For this review, take the finished solid that the model builds, in its own axes (mm). Face numbers are marked on the shaded views. A direction names the side the tool comes from. Round coordinates to 2 decimals unless told otherwise and drop trailing zeros. Write each loop counter-clockwise with the first axis right and the second up, starting at its lowest first coordinate (ties: lowest second). Pieces come first, ordered by that corner, then holes. Notation, with made-up numbers: (3, 49) - (16, 49) arc R24 cw to (16, 88) - close; hole circle Ø4 at (-9, 67.25). An arc over 180 degrees is marked (long way). One line per item, written item: value. Start each with the question number.
Q1. Mouldability with a two-part tool opening along Z and no side actions: class the marked faces 6, 7 and 8 as +Z half, -Z half, draft (parallel to the pull), parting line (faces both ways), or undercut.
Q2. Clearance check with flat-ended pins moving along their axes: pin 1 Ø4 at (x, z) = (3.5, 7) entering from -Y; pin 2 Ø3 at (y, z) = (1, 0) entering from -X; pin 3 Ø2 at (y, z) = (-5, -2.5) entering from +X. State where each tip first meets the part, or that it passes through.
Q3. Tool access review of the marked faces 1, 2, 3, 4 and 5: name each direction out of +Z, -Z, +X, -X, +Y, -Y from which nothing blocks a thin tool from reaching the whole face with its end or side.
Q4. For probe 1 along X at (y, z) = (3, -0.25); probe 2 along X at (y, z) = (5.75, 5.25); probe 3 along X at (y, z) = (0.75, 4.25), list the stretches that pass through material, from the lowest coordinate up.
Q5. Add section B-B on x = 8.5. Write out the cut boundary in (y, z), and give its area (3 significant figures).
Q6. Add section C-C on y = -6.5. Write out the cut boundary in (x, z).
Q7. Add section D-D on z = 7.25. Write out the cut boundary in (x, y), and give its area (3 significant figures).
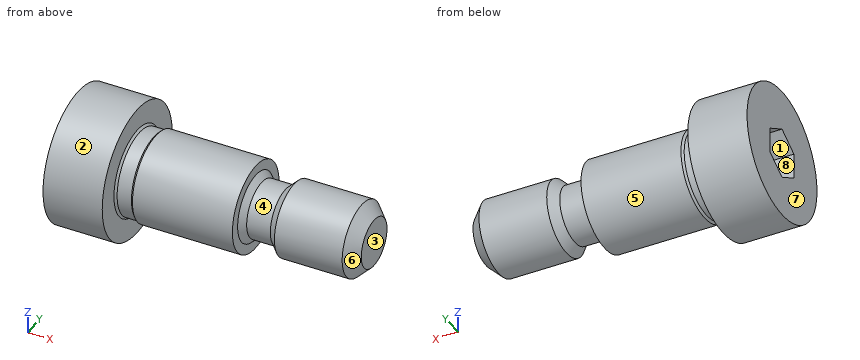
```python
from build123d import *

# Parameters (mm, degrees)
PROPERTYMANAGER_START         = -3
PROPERTYMANAGER_OUTLINE_R     = 5.71
PROPERTYMANAGER_DEPTH         = 19
PROPERTYMANAGER_START_2       = -8
PROPERTYMANAGER_2_OUTLINE_R   = 9
PROPERTYMANAGER_2_DEPTH       = 8
PROPERTYMANAGER_START_3       = 21.1549999
PROPERTYMANAGER_3_OUTLINE_R   = 5
PROPERTYMANAGER_3_DEPTH       = 9.1545
PROPERTYMANAGER_START_4       = 16
PROPERTYMANAGER_4_OUTLINE_R   = 3.845
PROPERTYMANAGER_4_DEPTH       = 14.3094999
PROPERTYMANAGER_START_5       = 2.4999999
PROPERTYMANAGER_5_OUTLINE_R   = 5.992
PROPERTYMANAGER_5_OUTLINE_R_2 = 5.71
PROPERTYMANAGER_5_DEPTH       = 13.5000001
HEXDRIVE_DEPTH                = 5


with BuildPart() as part:
    # PropertyManager: read off the stored shape, not the designer's step
    # PropertyManager outline → PropertyManager (new body)
    with BuildSketch(Plane.YZ.offset(PROPERTYMANAGER_START)):
        Circle(PROPERTYMANAGER_OUTLINE_R)
    extrude(amount=PROPERTYMANAGER_DEPTH)

    # PropertyManager 2 outline → PropertyManager 2 (add)
    with BuildSketch(Plane.YZ.offset(PROPERTYMANAGER_START_2)):
        Circle(PROPERTYMANAGER_2_OUTLINE_R)
        Polygon((0, 3.518949891), (3.0475, 1.759474945), (3.0475, -1.759474945), (0, -3.518949891), (-3.0475, -1.759474945), (-3.0475, 1.759474945), align=None, mode=Mode.SUBTRACT)
    extrude(amount=PROPERTYMANAGER_2_DEPTH)



with BuildPart() as body_2:
    # PropertyManager 3 outline → PropertyManager 3 (new body)
    with BuildSketch(Plane.YZ.offset(PROPERTYMANAGER_START_3)):
        Circle(PROPERTYMANAGER_3_OUTLINE_R)
    extrude(amount=PROPERTYMANAGER_3_DEPTH)


with BuildPart() as part_1:
    add(part.part)

    add(body_2.part)  # PropertyManager 4 merges body 2
    # PropertyManager 4 outline → PropertyManager 4 (add)
    with BuildSketch(Plane.YZ.offset(PROPERTYMANAGER_START_4)):
        Circle(PROPERTYMANAGER_4_OUTLINE_R)
    extrude(amount=PROPERTYMANAGER_4_DEPTH)

    # PropertyManager 5 outline → PropertyManager 5 (add)
    with BuildSketch(Plane.YZ.offset(PROPERTYMANAGER_START_5)):
        Circle(PROPERTYMANAGER_5_OUTLINE_R)
        Circle(PROPERTYMANAGER_5_OUTLINE_R_2, mode=Mode.SUBTRACT)
    extrude(amount=PROPERTYMANAGER_5_DEPTH)

    # PropertyManager 6 outline → PropertyManager 6 (revolve)
    with BuildSketch(Plane.YX):
        Polygon((3.3095, 32), (0, 32), (0, 30.3094999), (5, 30.30949995), align=None)
        Polygon((3.845, 21.1549999), (3.845, 20), (5, 21.15499995), align=None)
        Polygon((4.645, 16), (3.845, 16.8), (3.845, 16), align=None)
        Polygon((5.992, 2.4999999), (5.71, 2.4999999), (5.71, 2.218), align=None)
        Polygon((5.992, 0), (5.71, 0.282), (5.71, 0), align=None)
    revolve(axis=Axis((0, 0, 0), (1, 0, 0)))

    # BodySketch → BaseBody (revolve)
    with BuildSketch(Plane(origin=(0, 0, 0), x_dir=(1, 0, 0), z_dir=(0, 1, 0)), mode=Mode.PRIVATE) as basebody_sk:
        Polygon((0, 9), (-8, 9), (-8, 0), (32, 0), (32, 3.3095), (30.3095, 5), (21.155, 5), (20, 3.845), (16.8, 3.845), (16, 4.645), (16, 5.992), (2.5, 5.992), (2.218, 5.71), (0.282, 5.71), (0, 5.992), align=None)
    revolve(basebody_sk.sketch.rotate(Axis((-8, 0, 0), (1, 0, 0)), 180), axis=Axis((-8, 0, 0), (1, 0, 0)))

    # DriveSketch → HexDrive (cut)
    with BuildSketch(Plane.ZY.offset(8)):
        Polygon((3.518949891, 0), (1.759474945, 3.0475), (-1.759474945, 3.0475), (-3.518949891, 0), (-1.759474945, -3.0475), (1.759474945, -3.0475), align=None)
    extrude(amount=-HEXDRIVE_DEPTH, mode=Mode.SUBTRACT)


solid = part_1.part
```
Result set:
1. face 6: parting line
1. face 7: draft
1. face 8: undercut
2. pin 1: stops at y = -3.3
2. pin 2: stops at x = -3
2. pin 3: stops at x = 30.72
3. face 1: -X
3. face 2: +X, -X
3. face 3: +Z, -Z, +X, +Y, -Y
3. face 4: none
3. face 5: +X
4. probe 1: x = -3 to 32
4. probe 2: x = -8 to 0
4. probe 3: x = -8 to 16.33, 20.47 to 30.99
5. outline: circle Ø11.98 at (0, 0)
5. area: 113 mm^2
6. outline: (-8, -6.22) - (0, -6.22) - (0, 6.22) - (-8, 6.22) - close
7. outline: (-8, -5.33) - (0, -5.33) - (0, 5.33) - (-8, 5.33) - close
7. area: 85.3 mm^2
